```python
from build123d import *

# Parameters (mm, degrees)
SKETCH1_R           = 19.05
SKETCH1_W           = 152.4
SKETCH1_H           = 38.1
BOSS_EXTRUDE1_DEPTH = 25.4
SKETCH4_W           = 25.4
SKETCH4_H           = 38.1
BOSS_EXTRUDE3_DEPTH = 25.4
SKETCH6_W           = 25.4
SKETCH6_H           = 38.1
BOSS_EXTRUDE4_DEPTH = 25.4
SKETCH5_R           = 6.985
SKETCH5_R_2         = 1.905
CUT_EXTRUDE1_DEPTH  = 25.4
SKETCH7_W           = 50.8
SKETCH7_H           = 25.4
CUT_EXTRUDE2_DEPTH  = 25.4
SKETCH8_W           = 40.64
SKETCH8_H           = 20.32
CUT_EXTRUDE3_DEPTH  = 23.400004
SKETCH9_W           = 8.89
SKETCH9_H           = 20.32
CUT_EXTRUDE4_DEPTH  = 14.800072
SKETCH10_W          = 8.89
SKETCH10_H          = 2.54
CUT_EXTRUDE5_DEPTH  = 8.599932
SKETCH11_R          = 3.175
CUT_EXTRUDE6_DEPTH  = 110.617995785


with BuildPart() as part:
    # Sketch1 → Boss-Extrude1 (new body)
    with BuildSketch(Plane.XY):
        with Locations((76.2, 0)):
            Circle(SKETCH1_R)
        Rectangle(SKETCH1_W, SKETCH1_H)
    extrude(amount=BOSS_EXTRUDE1_DEPTH)

    # Sketch4 → Boss-Extrude3 (add)
    with BuildSketch(Plane.XY.offset(25.4)):
        with Locations((-63.5, 0)):
            Rectangle(SKETCH4_W, SKETCH4_H)
    extrude(amount=BOSS_EXTRUDE3_DEPTH)

    # Sketch6 → Boss-Extrude4 (add)
    with BuildSketch(Plane(origin=(0, 0, 0), x_dir=(-1, 0, 0), z_dir=(0, 0, -1))):
        with Locations((63.5, 0)):
            Rectangle(SKETCH6_W, SKETCH6_H)
    extrude(amount=BOSS_EXTRUDE4_DEPTH)

    # Sketch5 → Cut-Extrude1 (cut)
    with BuildSketch(Plane.ZY.offset(76.2)):
        with Locations((25.4, 0)):
            Circle(SKETCH5_R)
        with Locations((39.900098, 4.99999)):
            Circle(SKETCH5_R_2)
        with Locations((-9.099804, 4.99999)):
            Circle(SKETCH5_R_2)
        with Locations(Location((-9.099804, -4.99999, 0), (0, 0, 270))):
            Circle(SKETCH5_R_2)
        with Locations(Location((39.900098, -4.99999, 0), (0, 0, 270))):
            Circle(SKETCH5_R_2)
    extrude(amount=-CUT_EXTRUDE1_DEPTH, mode=Mode.SUBTRACT)

    # Sketch7 → Cut-Extrude2 (cut)
    with BuildSketch(Plane.XY.offset(25.4)):
        with Locations((-25.4, 0)):
            Rectangle(SKETCH7_W, SKETCH7_H)
    extrude(amount=-CUT_EXTRUDE2_DEPTH, mode=Mode.SUBTRACT)

    # Sketch8 → Cut-Extrude3 (cut)
    with BuildSketch(Plane(origin=(-50.8, 0, 0), x_dir=(0, 0, -1), z_dir=(1, 0, 0))):
        with Locations((-15.400147, 0)):
            Rectangle(SKETCH8_W, SKETCH8_H)
    extrude(amount=-CUT_EXTRUDE3_DEPTH, mode=Mode.SUBTRACT)

    # Sketch9 → Cut-Extrude4 (cut)
    with BuildSketch(Plane(origin=(-50.8, 0, 0), x_dir=(0, 0, -1), z_dir=(1, 0, 0))):
        with Locations((-40.165147, 0)):
            Rectangle(SKETCH9_W, SKETCH9_H)
        with Locations((9.364853, 0)):
            Rectangle(SKETCH9_W, SKETCH9_H)
    extrude(amount=-CUT_EXTRUDE4_DEPTH, mode=Mode.SUBTRACT)

    # Sketch10 → Cut-Extrude5 (cut)
    with BuildSketch(Plane(origin=(-65.600072, 0, 0), x_dir=(0, 0, -1), z_dir=(1, 0, 0))):
        with Locations((-40.165147, 0)):
            Rectangle(SKETCH10_W, SKETCH10_H)
        with Locations((9.364853, 0)):
            Rectangle(SKETCH10_W, SKETCH10_H)
    extrude(amount=-CUT_EXTRUDE5_DEPTH, mode=Mode.SUBTRACT)

    # Sketch11 → Cut-Extrude6 (cut, through all)
    with BuildSketch(Plane.XY.offset(25.4)):
        with Locations((76.2, 0)):
            Circle(SKETCH11_R)
    extrude(amount=-CUT_EXTRUDE6_DEPTH, mode=Mode.SUBTRACT)


solid = part.part
```
Input: part model. Units: mm. Frame: model coordinates. A direction names the side the tool comes from. Give positions to 0.01 mm unless a question says otherwise; leave off trailing zeros. Order: outer loops, then holes, each group sorted by start corner. A loop starts at its lowest first (then second) coordinate and runs counter-clockwise, first axis right, second up. Notation, with made-up numbers: (6.25, -39) -> (21.25, -39) arc R20 cw to (21.25, -32) -> close; hole circle Ø2 at (56.5, 26.25). An arc over 180 degrees is marked (long way). Write each question's results on one line, items separated by ' | '. Start each with the question number.
Item 1: Cut plane C-C on x = 22.5. Return the cut outline in (y, z), then the cut area to 3 significant figures.
Item 2: Contact query for flat-ended pins moving along their axis: P1, Ø8.5, axis at x = 76.2, y = 0, coming from the -Z side; P2, Ø22.5, axis at y = 0, z = 25.4, coming from the +X side; P3, Ø2, axis at y = -7, z = -8, coming from the +X side; P4, Ø4, axis at x = -50.5, y = 7.5, coming from the +Z side. Output: stop coordinate, or through.
Item 3: Set-up query: faces 1 (the flat face through (-26, 12.7, 13)), 2 (the flat face through (-62, -10.16, 16)), 3 (the cylindrical face through (-75.21, 0.31, 18.42)), 4 (the flat face through (-70, 6, 35.72)). Return all of +Z, -Z, +X, -X, +Y, -Y with unobstructed straight access to the full face (end or side cutting, diameter ignored); none if empty.
Item 4: Mould query, pull axis Z, two halves, no side actions, for faces 5 (the flat face through (-70, -6, 35.72)), 6 (the flat face through (-63, 0, -25.4)), 7 (the flat face through (0, 0, 13)), 8 (the flat face through (-64, 0, 50.8)). Classes: pulls with the +Z half, pulls with the -Z half, needs draft (parallel to the pull), parting line crosses it, or undercut.
Item 5: Line query: line 1 (Y direction, x = -75, z = 25); line 2 (Y direction, x = -24.5, z = 14); line 3 (X direction, y = 1.5, z = 1). Output: solid intervals per line, ascending.
Item 6: Cut plane A-A on x = -52.5. Return the cut outline in (y, z), then the cut area to 3 significant figures.
Item 7: Cut plane B-B on z = 30. Return the cut outline in (x, y).
Established:
1) outline: (-19.05, 0) -> (19.05, 0) -> (19.05, 25.4) -> (-19.05, 25.4) -> close | area: 968 mm^2
2) P1: z = 0 | P2: x = 95.25 | P3: x = -65.6 | P4: z = 50.8
3) face 1: +Z, -Z | face 2: none | face 3: -X | face 4: +X
4) face 5: undercut | face 6: pulls with the -Z half | face 7: needs draft | face 8: pulls with the +Z half
5) line 1: -19.05 to -6.97, 6.97 to 19.05 | line 2: -19.05 to -12.7, 12.7 to 19.05 | line 3: -76.2 to -74.2, 0 to 73.4, 79 to 95.19
6) outline: (-19.05, -25.4) -> (19.05, -25.4) -> (19.05, 50.8) -> (-19.05, 50.8) -> close; hole (-10.16, -13.81) -> (10.16, -13.81) -> (10.16, 44.61) -> (-10.16, 44.61) -> close | area: 1,720 mm^2
7) outline: (-76.2, -19.05) -> (-50.8, -19.05) -> (-50.8, -10.16) -> (-74.2, -10.16) -> (-74.2, -5.26) -> (-76.2, -5.26) -> close; (-76.2, 5.26) -> (-74.2, 5.26) -> (-74.2, 10.16) -> (-50.8, 10.16) -> (-50.8, 19.05) -> (-76.2, 19.05) -> close
